Autodesk Fusion 360 part; units mm, degrees
sketch "Sketch1" plane through (0, 0, 0) normal (0, 0, 1) x (1, 0, 0)
  line L0 (160, -190) -> (-160, -190)
  line L1 (-160, -190) -> (-160, 190)
  line L2 (-160, 190) -> (160, 190)
  line L3 (160, 190) -> (160, -190)
  line L4 (160, -190) -> (-160, 190) construction
  line L5 (-160, -190) -> (160, 190) construction
  dimension "d1" = 320
  dimension "d2" = 380
extrude "Extrude1" add sketch "Sketch1" along normal blind 25
sketch "Sketch2" plane through (0, 0, 25) normal (0, 0, 1) x (1, 0, 0)
  line L0 (160, 190) -> (-160, 190)
  line L1 (-160, 190) -> (-160, -190)
  line L2 (-160, -190) -> (160, -190)
  line L3 (160, -190) -> (160, 190)
  line L4 (-160, 190) -> (-125, 190)
  line L5 (-125, 190) -> (-125, 170)
  line L6 (-125, 170) -> (-160, 170)
  line L7 (-160, 170) -> (-160, 190)
  line L8 (160, 190) -> (125, 190)
  line L9 (125, 190) -> (125, 170)
  line L10 (125, 170) -> (160, 170)
  line L11 (160, 170) -> (160, 190)
  line L12 (160, -190) -> (125, -190)
  line L13 (125, -190) -> (125, -170)
  line L14 (125, -170) -> (160, -170)
  line L15 (160, -170) -> (160, -190)
  line L16 (-160, -190) -> (-125, -190)
  line L17 (-125, -190) -> (-125, -170)
  line L18 (-125, -170) -> (-160, -170)
  line L19 (-160, -170) -> (-160, -190)
  dimension "d5" = 35
  dimension "d6" = 20
  dimension "d7" = 35
  dimension "d8" = 20
  dimension "d9" = 20
  dimension "d10" = 35
  dimension "d11" = 35
  dimension "d12" = 20
hole "Hole1" at (-125, 170, 25) at (125, 170, 25) at (125, -170, 25) at (-125, -170, 25) direction (0, 0, -1) diameter 30 depth 25 tip angle 118
hole "Hole2" at (0, 0, 25) direction (0, 0, -1) diameter 40 depth 50 tip angle 118 counterbore diameter 70 counterbore depth 12
Can you work these out from the model? Positions are in its coordinate system, mm. A direction names the side the tool comes from. Give positions to 0.01 mm unless a question says otherwise; leave off trailing zeros. Loops run counter-clockwise (first coordinate to the right, second up) from the corner with the lowest first, then second, coordinate; pieces in that order, holes last. Notation, with made-up numbers: M 17,79.25 L 27,79.25 A24 cw 27,94.25 Z; hole C -32.5,78 d1. An arc over 180 degrees is marked long. One line per item, written item: value. Start each with the question number.
1) If we section it at D-D, the plane z = 3.75: Write out the boundary of the cut face in (x, y).
2) On a 3-axis mill with a long thin cutter (end or side, diameter ignored), from which of +Z, -Z, +X, -X, +Y, -Y can I reach the whole of each face in a straight line? I mean faces 4 (the face through (21, 28, 19)), 5 (the face through (-125.66, -155.015, 12.325)). Say none if no direction works.
3) If I drill on line 1 (X direction, y = 170, z = 7); line 2 (Y direction, x = -125, z = 12.75); line 3 (Y direction, x = 0, z = 20.75), over which ranges is the centre line in solid material (lowest first)? Write a range as [from, to].
4) Thinking about a two-plate mould opening in X: for faces 1 (the face through (160, 3, 12)), 2 (the face through (2, -190, 12)), 3 (the face through (124.34, 184.985, 12.325)), which applies, +X half, -X half, draft (parallel to the pull), parting line (faces both ways), or undercut?
5) If we section it at C-C, the plane y = 0: Write out the boundary of the cut face in (x, z).
6) If we section it at B-B, the plane x = 0: Write out the boundary of the cut face in (y, z).
7) If we section it at A-A, the plane y = 170: Write out the boundary of the cut face in (x, z), and give its area (3 significant figures).
Completed:
1. outline: M -160,-190 L 160,-190 L 160,190 L -160,190 Z; hole C -125,-170 d30; hole C -125,170 d30; hole C 0,0 d40; hole C 125,-170 d30; hole C 125,170 d30
2. face 4: +Z
2. face 5: +Z, -Z
3. line 1: x = [-160, -140], [-110, 110], [140, 160]
3. line 2: y = [-190, -185], [-155, 155], [185, 190]
3. line 3: y = [-190, -35], [35, 190]
4. face 1: +X half
4. face 2: draft
4. face 3: undercut
5. outline: M -160,0 L -20,0 L -20,13 L -35,13 L -35,25 L -160,25 Z; M 20,0 L 160,0 L 160,25 L 35,25 L 35,13 L 20,13 Z
6. outline: M -190,0 L -20,0 L -20,13 L -35,13 L -35,25 L -190,25 Z; M 20,0 L 190,0 L 190,25 L 35,25 L 35,13 L 20,13 Z
7. outline: M -160,0 L -140,0 L -140,25 L -160,25 Z; M -110,0 L 110,0 L 110,25 L -110,25 Z; M 140,0 L 160,0 L 160,25 L 140,25 Z
7. area: 6,500 mm^2
